Source: CAD feature listing. Evaluate the final solid. Frame: model axes, mm. A direction names the side the tool comes from. Round coordinates to 2 decimals unless told otherwise and drop trailing zeros. Order: outer loops, then holes, each group sorted by start corner. A loop starts at its lowest first (then second) coordinate and runs counter-clockwise, first axis right, second up. Notation, with made-up numbers: (71, 14.5) - (77, 14.5) arc R12 cw to (77, 29.5) - close; hole circle Ø4 at (26.25, 7.25). An arc over 180 degrees is marked (long way). Put each result on its own line as item: value. Start each with the question number.
1) Section C-C on z = -14.5. Output: boundary loops of the cut face in (x, y) (1 decimal), then the cut area to 3 significant figures.
2) Access query for faces 1 (the face through (-1.72, 7.75, -9.02)), 2 (the face through (0, 0, 9.525)). Directions: +Z, -Z, +X, -X, +Y, -Y. A direction counts if a zero-diameter tool reaches every point of the face in a straight line with its end or side. Return the directions, or none.
3) Line query: probe 1 along Y at (x, z) = (0.25, -17.25); probe 2 along Z at (x, y) = (-8.75, -7) (3 decimals); probe 3 along Y at (x, z) = (11, 5.25). Output: solid intervals per line, ascending. Write a range as [from, to].
4) Contact query for flat-ended pins moving along their axis: P1, Ø4, axis at x = -8, z = -0.5, coming from the +Y side; P2, Ø10, axis at y = -10, z = 0.5, coming from the +X side; P3, Ø2, axis at x = -5.5, z = -14, coming from the +Y side. Output: stop coordinate, or through.
5) Section A-A on x = -10. Output: boundary loops of the cut face in (y, z) (3 decimals), then the cut area to 3 significant figures.
```python
from build123d import *

# Parameters (mm, degrees)
F1_DEPTH = 9.525
F2_R     = 7.9375
F3_DEPTH = 19.05
F4_SIZE2 = 0.762
F4_SIZE  = 0.762


with BuildPart() as f1:
    # F0 (on Top) → F1 (new body)
    with BuildSketch(Plane.XY):
        with BuildLine():
            ThreePointArc((12.4640951626, 2.4364588605), (12.6408862143, 1.2239263531), (12.7, 0))
            ThreePointArc((12.7, 0), (11.559292099, -5.2604910579), (8.3420840677, -9.5759925547))
            Line((8.3420840677, -9.5759925547), (13.8707859253, -4.7596881355))
            Line((13.8707859253, -4.7596881355), (12.4640951626, 2.4364588605))
        make_face()
        with BuildLine():
            Line((2.8133821232, -14.3922970495), (8.3420840677, -9.5759925547))
            ThreePointArc((8.3420840677, -9.5759925547), (2.4364604633, -12.4640948492), (-4.1220107511, -12.0124530121))
            Line((-4.1220107511, -12.0124530121), (2.8133821232, -14.3922970495))
        make_face()
        with BuildLine():
            ThreePointArc((4.1220108652, 12.0124529729), (9.5759931131, 8.3420834267), (12.4640951626, 2.4364588605))
            Line((12.4640951626, 2.4364588605), (11.0574038021, 9.632608914))
            Line((11.0574038021, 9.632608914), (4.1220108652, 12.0124529729))
        make_face()
        with BuildLine():
            ThreePointArc((-12.4640951419, -2.4364589661), (-12.0124527553, 4.1220114996), (-8.3420840651, 9.5759925569))
            Line((-8.3420840651, 9.5759925569), (-13.8707859253, 4.7596881355))
            Line((-13.8707859253, 4.7596881355), (-12.4640951419, -2.4364589661))
        make_face()
        with BuildLine():
            Line((-11.0574038021, -9.632608914), (-4.1220107511, -12.0124530121))
            ThreePointArc((-4.1220107511, -12.0124530121), (-9.5759930381, -8.3420835128), (-12.4640951419, -2.4364589661))
            Line((-12.4640951419, -2.4364589661), (-11.0574038021, -9.632608914))
        make_face()
        with BuildLine():
            ThreePointArc((-8.3420840651, 9.5759925569), (-2.4364604025, 12.4640948611), (4.1220108652, 12.0124529729))
            Line((4.1220108652, 12.0124529729), (-2.8133821232, 14.3922970495))
            Line((-2.8133821232, 14.3922970495), (-8.3420840651, 9.5759925569))
        make_face()
        with BuildLine():
            ThreePointArc((8.3420840677, -9.5759925547), (11.559292099, -5.2604910579), (12.7, 0))
            ThreePointArc((12.7, 0), (12.6408862143, 1.2239263531), (12.4640951626, 2.4364588605))
            ThreePointArc((12.4640951626, 2.4364588605), (9.5759931131, 8.3420834267), (4.1220108652, 12.0124529729))
            ThreePointArc((4.1220108652, 12.0124529729), (-2.4364604025, 12.4640948611), (-8.3420840651, 9.5759925569))
            ThreePointArc((-8.3420840651, 9.5759925569), (-12.0124527553, 4.1220114996), (-12.4640951419, -2.4364589661))
            ThreePointArc((-12.4640951419, -2.4364589661), (-9.5759930381, -8.3420835128), (-4.1220107511, -12.0124530121))
            ThreePointArc((-4.1220107511, -12.0124530121), (2.4364604633, -12.4640948492), (8.3420840677, -9.5759925547))
        make_face()
    extrude(amount=F1_DEPTH)

    # F2 (on face) → F3 (join)
    with BuildSketch(Plane(origin=(0, 0, 0), x_dir=(1, 0, 0), z_dir=(0, 0, -1))):
        Circle(F2_R)
    extrude(amount=F3_DEPTH)

    # F4
    f4_edges = [f1.edges().sort_by_distance(p)[0] for p in [
        (4.122011, 12.012453, 9.525),
        (12.464095, 2.43646, 9.525),
        (8.342084, -9.575993, 9.525),
        (-12.464095, -2.43646, 9.525),
        (-4.122011, -12.012453, 9.525),
        (-8.342084, 9.575993, 9.525),
        (-7.9375, 0, -19.05),
        (8.342084, -9.575993, 0),
        (12.464095, 2.43646, 0),
        (4.122011, 12.012453, 0),
        (-8.342084, 9.575993, 0),
        (-12.464095, -2.43646, 0),
        (-4.122011, -12.012453, 0),
    ]]
    chamfer(f4_edges, length=F4_SIZE, length2=F4_SIZE2)


solid = f1.part
```
Answer sheet:
1. outline: circle Ø15.9 at (0, 0)
1. area: 198 mm^2
2. face 1: -Z
2. face 2: +Z, +X, -X, +Y, -Y
3. probe 1: [-7.93, 7.93]
3. probe 2: [0, 9.525]
3. probe 3: [-7.26, 9.65]
4. P1: y = 11.23
4. P2: x = 13.59
4. P3: y = 6.54
5. outline: (-9.995, 0.762) - (-9.19, 0) - (7.121, 0) - (8.132, 0.762) - (8.132, 8.763) - (7.121, 9.525) - (-9.19, 9.525) - (-9.995, 8.763) - close
5. area: 171 mm^2
